Geometry check sheet. Reference: drawing and pictorial views, mm from the part's lowest x, y, z. A direction names the side the tool comes from. Round coordinates to 2 decimals unless told otherwise and drop trailing zeros. Loops run counter-clockwise (first coordinate to the right, second up) from the corner with the lowest first, then second, coordinate; pieces in that order, holes last. Notation, with made-up numbers: (7.25, -5) - (35.25, -5) arc R17 ccw to (35.25, 19) - close; hole circle Ø4 at (-3.75, 27.25). An arc over 180 degrees is marked (long way). Put each result on its own line as item: value. Start each with the question number.
Item 1: Section check C-C, the plane y = 22.5. Record the cut outline in (x, z) (1 decimal), and give its area (3 significant figures).
Item 2: Section check A-A, the plane y = 29. Record the cut outline in (x, z).
Item 3: Material ranges on line 1 along Y through (x, z) = (29, 10); line 2 along X through (y, z) = (48, 3.75) (1 decimal); line 3 along X through (y, z) = (28, 13.75) (1 decimal), recorded low to high.
Item 4: Gauge pin test, flat ends, axial feed: pin 1 Ø1.5 at (x, y) = (42.5, 23.5) entering from -Z; pin 2 Ø7.5 at (x, z) = (42, 6) entering from -Y (1 decimal); pin 3 Ø3 at (x, z) = (13.5, 9) entering from -Y; pin 4 Ø8 at (x, z) = (20, 7.5) entering from +Y (1 decimal). Record the tip position at first contact, or that the pin passes through.
Item 5: Draft check along X on the marked faces 1, 2 and 3. Enter one of: pulls with the +X half, pulls with the -X half, needs draft (parallel to the pull), parting line crosses it, or undercut.
Item 6: Tool access check on the marked faces 4 and 5. Record the directions out of +Z, -Z, +X, -X, +Y, -Y that give a thin tool (end or side, any length) a straight path to the whole face; none if there is none.
Item 7: Section check D-D, the plane x = 17.5. Record the cut outline in (y, z) (1 decimal), and give its area (3 significant figures).
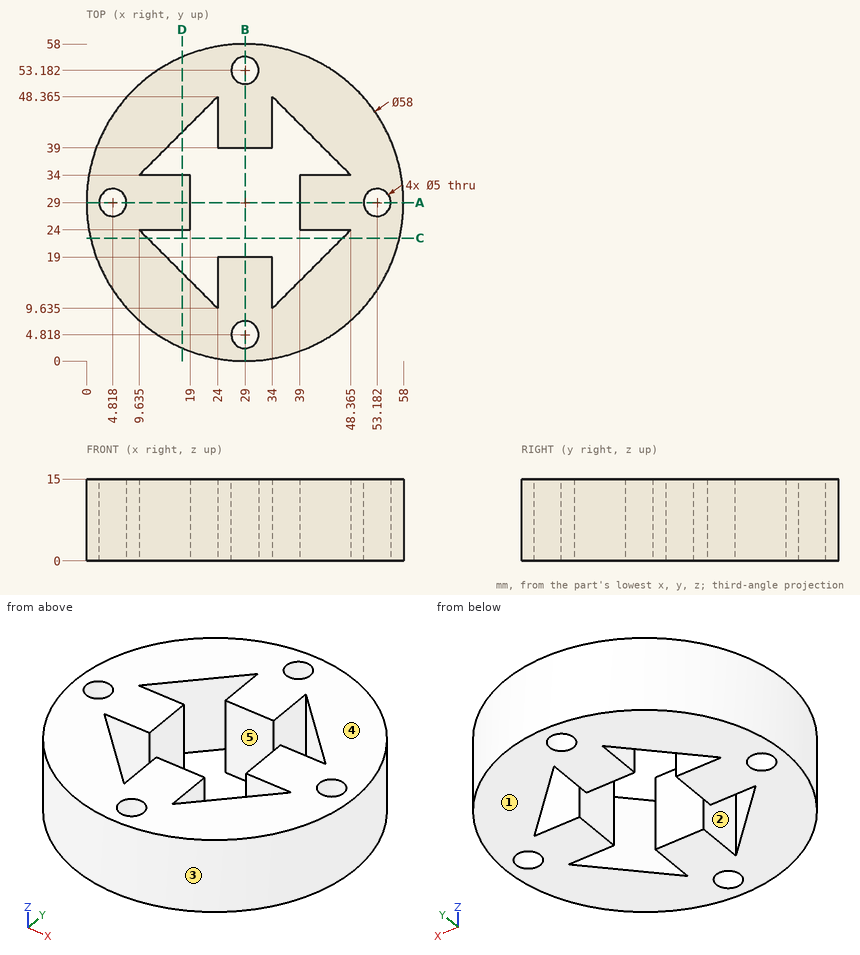
Check result:
1. outline: (0.7, 0) - (11.1, 0) - (11.1, 15) - (0.7, 15) - close; (46.9, 0) - (57.3, 0) - (57.3, 15) - (46.9, 15) - close
1. area: 312 mm²
2. outline: (0, 0) - (2.32, 0) - (2.32, 15) - (0, 15) - close; (7.32, 0) - (19, 0) - (19, 15) - (7.32, 15) - close; (39, 0) - (50.68, 0) - (50.68, 15) - (39, 15) - close; (55.68, 0) - (58, 0) - (58, 15) - (55.68, 15) - close
3. line 1: 0 to 2.32, 7.32 to 19, 39 to 50.68, 55.68 to 58
3. line 2: 7.1 to 23.6, 24 to 34, 34.4 to 50.9
3. line 3: 0 to 2.5, 7.1 to 19, 39 to 50.9, 55.5 to 58
4. pin 1: z = 0
4. pin 2: y = 1.5
4. pin 3: y = 3.6
4. pin 4: y = 57.6
5. face 1: needs draft
5. face 2: undercut
5. face 3: parting line crosses it
6. face 4: +Z, +X, -X, +Y, -Y
6. face 5: +Z, -Z
7. outline: (2.4, 0) - (16.1, 0) - (16.1, 15) - (2.4, 15) - close; (24, 0) - (34, 0) - (34, 15) - (24, 15) - close; (41.9, 0) - (55.6, 0) - (55.6, 15) - (41.9, 15) - close
7. area: 563 mm²
